For this review, take the finished solid that the model builds, in its own axes (mm). A direction names the side the tool comes from. Round coordinates to 2 decimals unless told otherwise and drop trailing zeros. Write each loop counter-clockwise with the first axis right and the second up, starting at its lowest first coordinate (ties: lowest second). Pieces come first, ordered by that corner, then holes. Notation, with made-up numbers: M 28,80.5 L 72,80.5 A31 ccw 72,117.5 Z; hole C 1.5,-11 d7. An arc over 180 degrees is marked long. Answer in a Markdown table with one row per item.
```python
from build123d import *

# Parameters (mm, degrees)
SKETCH2_W                = 200
SKETCH2_H                = 150
BOSS_EXTRUDE1_DEPTH      = 80
FILLET1_R                = 10
SHELL1_T                 = -2
SHELL1_THICKNESS_2_DEPTH = 13
SKETCH5_W                = 36.5
SKETCH5_H                = 27.5
CUT_EXTRUDE1_DEPTH       = 2
BOSS_EXTRUDE2_DEPTH      = 16
SKETCH7_W                = 36.5
SKETCH7_H                = 27.5
CUT_EXTRUDE2_DEPTH       = 2
BOSS_EXTRUDE3_DEPTH      = 16
SKETCH10_W               = 36.5
SKETCH10_H               = 27.5
CUT_EXTRUDE4_DEPTH       = 2
BOSS_EXTRUDE4_DEPTH      = 16
SKETCH13_W               = 38
SKETCH13_H               = 19.1
CUT_EXTRUDE5_DEPTH       = 2
BOSS_EXTRUDE5_DEPTH      = 13.5
SKETCH15_W               = 10.5
SKETCH15_H               = 9.367949192
CUT_EXTRUDE6_DEPTH       = 3
CUT_EXTRUDE8_REACH       = 150.408
SKETCH20_R               = 8


with BuildPart() as part:
    # Sketch2 → Boss-Extrude1 (new body)
    with BuildSketch(Plane(origin=(0, 0, 0), x_dir=(1, 0, 0), z_dir=(0, 1, 0))):
        Rectangle(SKETCH2_W, SKETCH2_H)
    extrude(amount=BOSS_EXTRUDE1_DEPTH)

    # Fillet1
    fillet1_edges = [part.edges().sort_by_distance(p)[0] for p in [
        (100, 40, 75),
        (-100, 40, 75),
        (-100, 40, -75),
        (100, 40, -75),
    ]]
    fillet(fillet1_edges, radius=FILLET1_R)

    # Shell1
    shell1_openings = [part.faces().sort_by_distance(p)[0] for p in [
        (0, 80, 0),
    ]]
    offset(amount=SHELL1_T, openings=shell1_openings, kind=Kind.INTERSECTION)

    # Shell1 thickness 2 face (on inner face of the shell) → Shell1 thickness 2 (add)
    with BuildSketch(Plane(origin=(0, 2, 0), x_dir=(0, 0, -1), z_dir=(0, -1, 0))):
        with BuildLine():
            ThreePointArc((73, -90), (70.656854249, -95.656854249), (65, -98))
            Line((65, -98), (-65, -98))
            ThreePointArc((-65, -98), (-70.656854249, -95.656854249), (-73, -90))
            Line((-73, -90), (-73, 90))
            ThreePointArc((-73, 90), (-70.656854249, 95.656854249), (-65, 98))
            Line((-65, 98), (65, 98))
            ThreePointArc((65, 98), (70.656854249, 95.656854249), (73, 90))
            Line((73, 90), (73, -90))
        make_face()
    extrude(amount=-SHELL1_THICKNESS_2_DEPTH)

    # Sketch5 → Cut-Extrude1 (cut)
    with BuildSketch(Plane.XY.offset(75)):
        with Locations((0, 30.75)):
            Rectangle(SKETCH5_W, SKETCH5_H)
        Polygon((-18.25, 43.5), (-19.75, 44.366025404), (-19.75, 41.633974596), (-18.25, 42.5), align=None)
        Polygon((-19.75, 19.866025404), (-18.25, 19), (-18.25, 18), (-19.75, 17.133974596), align=None)
        Polygon((19.75, 17.133974596), (19.75, 19.866025404), (18.25, 19), (18.25, 18), align=None)
        Polygon((19.75, 41.633974596), (18.25, 42.5), (18.25, 43.5), (19.75, 44.366025404), align=None)
    extrude(amount=-CUT_EXTRUDE1_DEPTH, mode=Mode.SUBTRACT)

    # Sketch6 → Boss-Extrude2 (add)
    with BuildSketch(Plane(origin=(0, 0, 73), x_dir=(-1, 0, 0), z_dir=(0, 0, -1))):
        Polygon((18.25, 15), (21.25, 15), (21.25, 47.5), (18.25, 47.5), (18.25, 43.5), (19.75, 44.366025404), (19.75, 41.633974596), (18.25, 42.5), (18.25, 19), (19.75, 19.866025404), (19.75, 17.133974596), (18.25, 18), align=None)
        Polygon((-21.25, 47.5), (-21.25, 15), (-18.25, 15), (-18.25, 18), (-19.75, 17.133974596), (-19.75, 19.866025404), (-18.25, 19), (-18.25, 42.5), (-19.75, 41.633974596), (-19.75, 44.366025404), (-18.25, 43.5), (-18.25, 47.5), align=None)
    extrude(amount=BOSS_EXTRUDE2_DEPTH)

    # Sketch7 → Cut-Extrude2 (cut)
    with BuildSketch(Plane(origin=(100, 0, 0), x_dir=(0, 0, -1), z_dir=(1, 0, 0))):
        with Locations((0, 30.75)):
            Rectangle(SKETCH7_W, SKETCH7_H)
        Polygon((-18.25, 43.5), (-19.75, 44.366025404), (-19.75, 41.633974596), (-18.25, 42.5), align=None)
        Polygon((-19.75, 19.866025404), (-18.25, 19), (-18.25, 18), (-19.75, 17.133974596), align=None)
        Polygon((19.75, 17.133974596), (19.75, 19.866025404), (18.25, 19), (18.25, 18), align=None)
        Polygon((19.75, 41.633974596), (18.25, 42.5), (18.25, 43.5), (19.75, 44.366025404), align=None)
    extrude(amount=-CUT_EXTRUDE2_DEPTH, mode=Mode.SUBTRACT)

    # Sketch8 → Boss-Extrude3 (add)
    with BuildSketch(Plane.ZY.offset(-98)):
        Polygon((-21.25, 47.5), (-18.25, 47.5), (-18.25, 43.5), (-19.75, 44.366025404), (-19.75, 41.633974596), (-18.25, 42.5), (-18.25, 19), (-19.75, 19.866025404), (-19.75, 17.133974596), (-18.25, 18), (-18.25, 15), (-21.25, 15), align=None)
        Polygon((19.75, 44.366025404), (18.25, 43.5), (18.25, 47.5), (21.25, 47.5), (21.25, 15), (18.25, 15), (18.25, 18), (19.75, 17.133974596), (19.75, 19.866025404), (18.25, 19), (18.25, 42.5), (19.75, 41.633974596), align=None)
    extrude(amount=BOSS_EXTRUDE3_DEPTH)

    # Sketch10 → Cut-Extrude4 (cut)
    with BuildSketch(Plane.ZY.offset(100)):
        with Locations((0, 30.75)):
            Rectangle(SKETCH10_W, SKETCH10_H)
        Polygon((-18.25, 43.5), (-19.75, 44.366025404), (-19.75, 41.633974596), (-18.25, 42.5), align=None)
        Polygon((-19.75, 19.866025404), (-18.25, 19), (-18.25, 18), (-19.75, 17.133974596), align=None)
        Polygon((19.75, 17.133974596), (19.75, 19.866025404), (18.25, 19), (18.25, 18), align=None)
        Polygon((19.75, 41.633974596), (18.25, 42.5), (18.25, 43.5), (19.75, 44.366025404), align=None)
    extrude(amount=-CUT_EXTRUDE4_DEPTH, mode=Mode.SUBTRACT)

    # Sketch11 → Boss-Extrude4 (add)
    with BuildSketch(Plane(origin=(-98, 0, 0), x_dir=(0, 0, -1), z_dir=(1, 0, 0))):
        Polygon((-18.25, 47.5), (-21.25, 47.5), (-21.25, 15), (-18.25, 15), (-18.25, 18), (-19.75, 17.133974596), (-19.75, 19.866025404), (-18.25, 19), (-18.25, 42.5), (-19.75, 41.633974596), (-19.75, 44.366025404), (-18.25, 43.5), align=None)
        Polygon((19.75, 44.366025404), (18.25, 43.5), (18.25, 47.5), (21.25, 47.5), (21.25, 15), (18.25, 15), (18.25, 18), (19.75, 17.133974596), (19.75, 19.866025404), (18.25, 19), (18.25, 42.5), (19.75, 41.633974596), align=None)
    extrude(amount=BOSS_EXTRUDE4_DEPTH)

    # Sketch13 → Cut-Extrude5 (cut)
    with BuildSketch(Plane.XY.offset(75)):
        Polygon((41, 39.3), (39.5, 40.166025404), (39.5, 37.433974596), (41, 38.3), align=None)
        with Locations((60, 30.75)):
            Rectangle(SKETCH13_W, SKETCH13_H)
        Polygon((41, 22.2), (39.5, 21.333974596), (39.5, 24.066025404), (41, 23.2), align=None)
        Polygon((79, 22.2), (79, 23.2), (80.5, 24.066025404), (80.5, 21.333974596), align=None)
        Polygon((79, 39.3), (80.5, 40.166025404), (80.5, 37.433974596), (79, 38.3), align=None)
    extrude(amount=-CUT_EXTRUDE5_DEPTH, mode=Mode.SUBTRACT)

    # Sketch14 → Boss-Extrude5 (add)
    with BuildSketch(Plane(origin=(0, 0, 73), x_dir=(-1, 0, 0), z_dir=(0, 0, -1))):
        Polygon((-79, 43.3), (-82, 43.3), (-82, 15), (-79, 15), (-79, 22.2), (-80.5, 21.333974596), (-80.5, 24.066025404), (-79, 23.2), (-79, 38.3), (-80.5, 37.433974596), (-80.5, 40.166025404), (-79, 39.3), align=None)
        Polygon((-39.5, 40.166025404), (-41, 39.3), (-41, 43.3), (-38, 43.3), (-38, 15), (-41, 15), (-41, 22.2), (-39.5, 21.333974596), (-39.5, 24.066025404), (-41, 23.2), (-41, 38.3), (-39.5, 37.433974596), align=None)
    extrude(amount=BOSS_EXTRUDE5_DEPTH)

    # Sketch15 → Cut-Extrude6 (cut)
    with BuildSketch(Plane.ZY.offset(-38)):
        with Locations((66.75, 30.75)):
            Rectangle(SKETCH15_W, SKETCH15_H)
    extrude(amount=-CUT_EXTRUDE6_DEPTH, mode=Mode.SUBTRACT)

    # Sketch18 → Cut-Revolve1 (revolve, cut)
    with BuildSketch(Plane(origin=(0, 0, 0), x_dir=(0, 0, -1), z_dir=(1, 0, 0)), mode=Mode.PRIVATE) as cut_revolve1_sk:
        Polygon((-42.5, 0), (-70, 0), (-47.5, 10), (-42.5, 10), align=None)
    revolve(cut_revolve1_sk.sketch.rotate(Axis((0, 0, 0), (0, 1, 0)), 180), axis=Axis((0, 0, 0), (0, 1, 0)), mode=Mode.SUBTRACT)

    # Cut-Extrude8: up to this face of the body (flat: up to its plane)
    cut_extrude8_end = Plane(part.part.faces().sort_by_distance((-0.172388952, 15, -0.411685035))[0])
    # Sketch20 → Cut-Extrude8 (cut, up to the picked face)
    with BuildSketch(Plane.XZ, mode=Mode.PRIVATE) as cut_extrude8_sk1:
        with Locations(Location((0, -42.5, 0), (0, 0, 270))):
            Circle(SKETCH20_R)
    cut_extrude8_tool1 = split(extrude(cut_extrude8_sk1.sketch, amount=-CUT_EXTRUDE8_REACH, mode=Mode.PRIVATE), bisect_by=cut_extrude8_end, keep=Keep.BOTH, mode=Mode.PRIVATE)
    add(cut_extrude8_tool1.solids().sort_by(Axis((0, 0, -42.5), (0, 1, 0)))[0], mode=Mode.SUBTRACT)


solid = part.part
```
Q1. Take a section at D-D (y = 32). State how many separate pieces and enclosed holes the cut face has, then the cut area to 3 significant figures.
Found:
| item | result |
|---|---|
| separate pieces | 5 |
| enclosed holes | 0 |
| area | 1,400 mm² |
Q2. Mouldability with a two-part tool opening along X and no side actions: class faces 4 (the face through (91, 46, -18.25)), 5 (the face through (-100, 48, 1)), 6 (the face through (-1, 0, 0)) as +X half, -X half, draft (parallel to the pull), parting line (faces both ways), or undercut.
Found:
| item | result |
|---|---|
| face 4 | undercut |
| face 5 | -X half |
| face 6 | draft |
Q3. For probe 1 along X at (y, z) = (58.5, -16); probe 2 along Z at (x, y) = (-89.5, 31.5); probe 3 along Z at (x, y) = (0, 11), list the stretches that pass through material, from the lowest coordinate up.
Found:
| item | result |
|---|---|
| probe 1 | -100 to -98, 98 to 100 |
| probe 2 | -75 to -73, -21.25 to -18.25, 18.25 to 21.25, 73 to 75 |
| probe 3 | -75 to -50.5, -34.5 to 75 |
Q4. Take a section at B-B (x = 0). State the section outline as (y, z) points.
Found:
| item | result |
|---|---|
| outline | M 0,-75 L 80,-75 L 80,-73 L 15,-73 L 15,-50.5 L 8.67,-50.5 L 0,-70 Z; M 0,-34.5 L 15,-34.5 L 15,73 L 17,73 L 17,75 L 0,75 L 0,70 L 10,47.5 L 10,42.5 L 0,42.5 Z; M 44.5,73 L 80,73 L 80,75 L 44.5,75 Z |
Q5. Take a section at A-A (z = 0). State the section outline as (x, y) points.
Found:
| item | result |
|---|---|
| outline | M -100,0 L -70,0 L -47.5,10 L -42.5,10 L -42.5,0 L 42.5,0 L 42.5,10 L 47.5,10 L 70,0 L 100,0 L 100,17 L 98,17 L 98,15 L -98,15 L -98,17 L -100,17 Z; M -100,44.5 L -98,44.5 L -98,80 L -100,80 Z; M 98,44.5 L 100,44.5 L 100,80 L 98,80 Z |
Q6. Insertion check: P1, Ø2.5, axis at x = 94.5, y = 16.5, coming from the +Z side; P2, Ø4.5, axis at y = 32, z = 68.5, coming from the +X side; P3, Ø2, axis at y = 42, z = 69.5, coming from the +X side. Each pin has a flat end and moves straight along its axis. Give the tip position at first contact, or say it passes through.
Found:
| item | result |
|---|---|
| P1 | z = 74.46 |
| P2 | x = 99.92 |
| P3 | x = 99.37 |
Q7. Take a section at C-C (y = 50). State the section outline as (x, z) points.
Found:
| item | result |
|---|---|
| outline | M -100,-65 A10 ccw -90,-75 L 90,-75 A10 ccw 100,-65 L 100,65 A10 ccw 90,75 L -90,75 A10 ccw -100,65 Z; hole M -98,-65 A8 ccw -90,-73 L 90,-73 A8 ccw 98,-65 L 98,65 A8 ccw 90,73 L -90,73 A8 ccw -98,65 Z |
Q8. Machinability: for faces 1 (the face through (-90, 31, -21.25)), 2 (the face through (41, 31, 73)), 3 (the face through (-3.7, 10, 42.5)), which of the approach directions +Z, -Z, +X, -X, +Y, -Y give a long, thin tool a straight path to every point of the face, cutting with its end or side? Answer none if there is none.
Found:
| item | result |
|---|---|
| face 1 | +Y |
| face 2 | +Z |
| face 3 | -Y |
